Check sheet for the modelled part. Datum: model origin and axes. Units: mm. Face numbers are marked on the shaded views. A direction names the side the tool comes from. Round coordinates to 2 decimals unless told otherwise and drop trailing zeros. Write each loop counter-clockwise with the first axis right and the second up, starting at its lowest first coordinate (ties: lowest second). Pieces come first, ordered by that corner, then holes.
Item 1: Section check C-C, the plane y = 49.5. Record the cut outline in (x, z), plus the area to 3 significant figures.
Item 2: Section check A-A, the plane z = -42. Record the cut outline in (x, y), plus the area to 3 significant figures.
Item 3: Depth check by flat-ended pin: pin 1 (1.5 mm diameter, centred on y = 17, z = 35, fed in from +X); pin 2 (6 mm diameter, centred on x = -34.5, y = 22, fed in from +Z); pin 3 (2 mm diameter, centred on y = 29.5, z = -2, fed in from +X). Enter the tip coordinate at first touch or a pass-through.
Item 4: Release check for a two-part mould opening along Z. For the marked faces 1, 2, 3 and 4 record: pulls with the +Z half, pulls with the -Z half, needs draft (parallel to the pull), parting line crosses it, or undercut.
Item 5: Section check D-D, the plane z = 44. Record the cut outline in (x, y), plus the area to 3 significant figures.
Item 6: Section check B-B, the plane x = 29. Record the cut outline in (y, z), plus the area to 3 significant figures.
Item 7: Set-up check for the marked faces 5 and 6: record each of +Z, -Z, +X, -X, +Y, -Y from which the full face is reachable in a straight line by a thin tool's end or side.
Item 8: Material ranges on line 1 along Z through (x, y) = (42.5, 46); line 2 along Z through (x, y) = (56, 29); line 3 along X through (y, z) = (53.5, -59), recorded low to high.
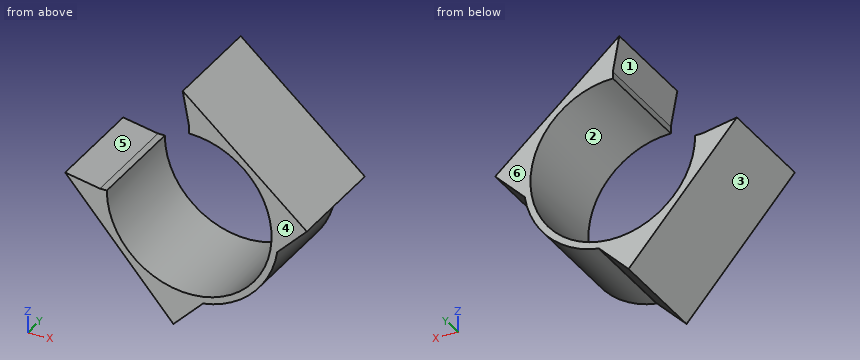
from build123d import *

# Parameters (mm, degrees)
BOSS_EXTRUDE1_DEPTH = 62
SKETCH3_W           = 15
SKETCH3_H           = 80.278098872
CUT_EXTRUDE1_DEPTH  = 24.5
SKETCH4_W           = 18.12750906
SKETCH4_H           = 69.709686178
CUT_EXTRUDE2_DEPTH  = 24.5


with BuildPart() as part:
    # Sketch1 → Boss-Extrude1 (new body)
    with BuildSketch(Plane(origin=(0, 0, 0), x_dir=(1, 0, 0), z_dir=(0, 1, 0))):
        with BuildLine():
            Line((-52.000074422, -0.000131195), (-48, -0.000131195))
            ThreePointArc((-48, -0.000131195), (33.941079112, 33.941171881), (0, -48))
            Line((0, -48), (0, -52.000074422))
            Line((0, -52.000074422), (-3.768119303, -72.286566827))
            Line((-3.768119303, -72.286566827), (68.579771311, -9.185198192))
            Line((68.579771311, -9.185198192), (75.652096433, -2.112870208))
            Line((75.652096433, -2.112870208), (58.450826977, 15.088392287))
            Line((58.450826977, 15.088392287), (51.378501856, 8.016064304))
            ThreePointArc((51.378501856, 8.016064304), (36.769597807, 36.769612685), (8.016043515, 51.378505099))
            Line((8.016043515, 51.378505099), (15.088368636, 58.450833083))
            Line((15.088368636, 58.450833083), (-2.112934166, 75.652128925))
            Line((-2.112934166, 75.652128925), (-9.185259288, 68.579800942))
            Line((-9.185259288, 68.579800942), (-72.286524075, -3.768180248))
            Line((-72.286524075, -3.768180248), (-52.000074422, -0.000131195))
        make_face()
    extrude(amount=BOSS_EXTRUDE1_DEPTH)

    # Sketch3 → Cut-Extrude1 (cut)
    with BuildSketch(Plane(origin=(38.882498626, 0, 38.882482893), x_dir=(0.707106638, 0, -0.707106924), z_dir=(0.707106924, 0, 0.707106638))):
        with Locations((49.498294294, 40.139049436)):
            Rectangle(SKETCH3_W, SKETCH3_H)
    extrude(amount=-CUT_EXTRUDE1_DEPTH, mode=Mode.SUBTRACT)

    # Sketch4 → Cut-Extrude2 (cut)
    with BuildSketch(Plane(origin=(-38.882531973, 0, -38.88251624), x_dir=(-0.707106638, 0, 0.707106924), z_dir=(-0.707106924, 0, -0.707106638))):
        with Locations((-51.062048824, 34.854843089)):
            Rectangle(SKETCH4_W, SKETCH4_H)
    extrude(amount=-CUT_EXTRUDE2_DEPTH, mode=Mode.SUBTRACT)


solid = part.part
Values found:
1. outline: (-72.29, 3.77) - (-9.19, -68.58) - (8.14, -51.26) - (8.23, -51.34) arc R52 ccw to (51.34, -8.23) - (51.26, -8.14) - (68.58, 9.19) - (-3.77, 72.29) - (0, 52) - (0, 48) arc R48 cw (long way) to (-48, 0) - (-52, 0) - close
1. area: 2,090 mm2
2. outline: (-32.37, 0) - (-23.24, 0) - (-23.24, 62) - (-32.37, 62) - close; (23.24, 0) - (30.66, 0) - (30.66, 62) - (23.24, 62) - close
2. area: 1,030 mm2
3. pin 1: stops at x = 39.84
3. pin 2: stops at z = -29.96
3. pin 3: stops at x = 58.39
4. face 1: undercut
4. face 2: undercut
4. face 3: pulls with the -Z half
4. face 4: needs draft
5. outline: (19.18, 0) - (28.66, 0) - (28.66, 62) - (19.18, 62) - close
5. area: 588 mm2
6. outline: (0, -43.16) - (62, -43.16) - (62, -38.25) - (0, -38.25) - close; (0, 38.25) - (62, 38.25) - (62, 43.71) - (0, 43.71) - close
6. area: 643 mm2
7. face 5: +Z, +Y, -Y
7. face 6: +Z, -Z, +X, -X, +Y
8. line 1: z = -29.96 to -22.31, 22.31 to 31.93
8. line 2: z = -3.39 to 20.16
8. line 3: x = -17.54 to 0.39
